Study the drawing (mm; zero at the part's minimum x, y, z) and answer. A direction names the side the tool comes from. Round coordinates to 2 decimals unless told otherwise and drop trailing zeros. Order: outer loops, then holes, each group sorted by start corner. A loop starts at its lowest first (then second) coordinate and runs counter-clockwise, first axis right, second up. Notation, with made-up numbers: (-36.75, 32) -> (-8.75, 32) arc R19 cw to (-8.75, 37) -> close; hole circle Ø9 at (62, 22). An arc over 180 degrees is marked (long way). Use one line per item in the form item = value.
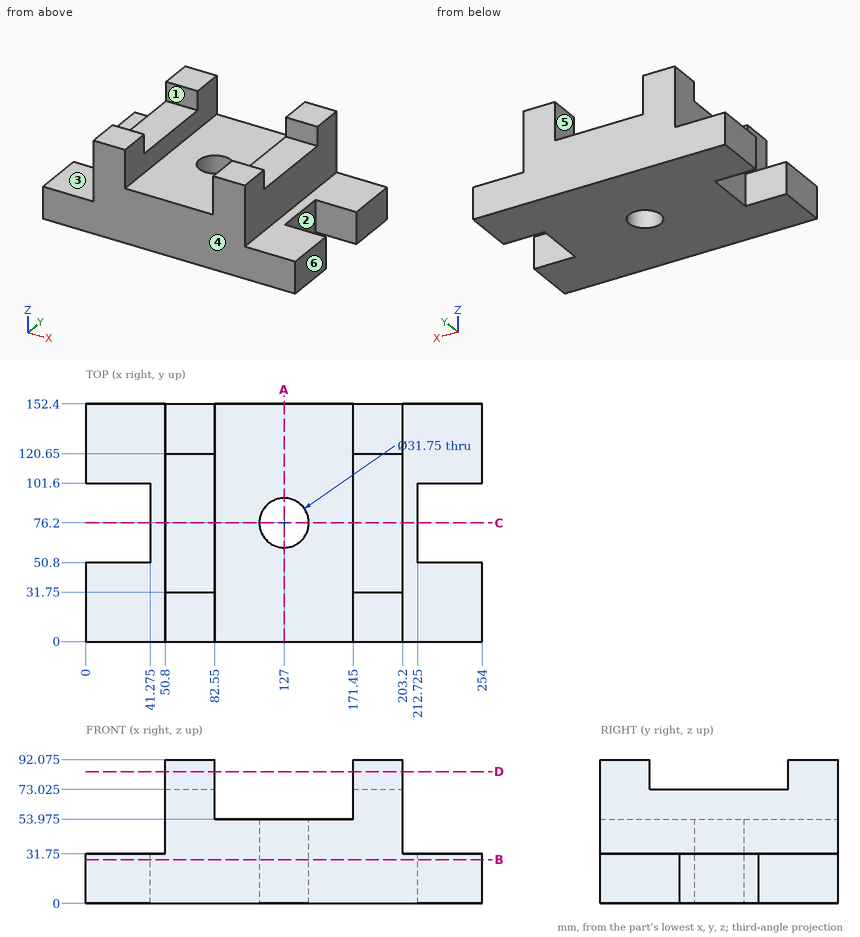
Item 1: Flat-ended cylindrical pins translate along their axes: P1, Ø1, axis at y = 120, z = 66.5, coming from the -X side; P2, Ø3, axis at x = 213.5, y = 68.5, coming from the -Z side; P3, Ø8, axis at y = 33.5, z = 81, coming from the +X side; P4, Ø5, axis at y = 77.5, z = 21, coming from the +X side (3 decimals). Find the tip coordinate at first contact, or state that the pin passes through.
Findings:
P1 = 50.8
P2 = 0
P3 = 203.2
P4 = 212.725
Item 2: For the marked faces 1, 2 and 3, determine the directions among +Z, -Z, +X, -X, +Y, -Y from which every point of the face is accessible in a straight line to the end or side of a thin tool.
Findings:
face_1 = +Z, +X, -X
face_2 = +Z, -Z, +X
face_3 = +Z, -X, +Y, -Y
Item 3: Consider line 1 along Y through (x, z) = (127, 38) (3 decimals); line 2 along X through (y, z) = (144.5, 62); line 3 along Y through (x, z) = (225.5, 26.5). Determine where each line is inside the solid, lowest interval first.
Findings:
line_1 = 0 to 60.325, 92.075 to 152.4
line_2 = 50.8 to 82.55, 171.45 to 203.2
line_3 = 0 to 50.8, 101.6 to 152.4
Item 4: The part is cut by section B-B, the plane z = 28. Give the vertices of the cut face in (x, y) (3 decimals).
Findings:
outline = (0, 0) -> (254, 0) -> (254, 50.8) -> (212.725, 50.8) -> (212.725, 101.6) -> (254, 101.6) -> (254, 152.4) -> (0, 152.4) -> (0, 101.6) -> (41.275, 101.6) -> (41.275, 50.8) -> (0, 50.8) -> close; hole circle Ø31.75 at (127, 76.2)
Item 5: The part is cut by section C-C, the plane y = 76.2. Give the vertices of the cut face in (x, z) (3 decimals), and give its area (3 significant figures).
Findings:
outline = (41.275, 0) -> (111.125, 0) -> (111.125, 53.975) -> (82.55, 53.975) -> (82.55, 73.025) -> (50.8, 73.025) -> (50.8, 31.75) -> (41.275, 31.75) -> close; (142.875, 0) -> (212.725, 0) -> (212.725, 31.75) -> (203.2, 31.75) -> (203.2, 73.025) -> (171.45, 73.025) -> (171.45, 53.975) -> (142.875, 53.975) -> close
area = 8,330 mm^2
Item 6: The part is cut by section D-D, the plane z = 84.5. Give the vertices of the cut face in (x, y), and give its area (3 significant figures).
Findings:
outline = (50.8, 0) -> (82.55, 0) -> (82.55, 31.75) -> (50.8, 31.75) -> close; (50.8, 120.65) -> (82.55, 120.65) -> (82.55, 152.4) -> (50.8, 152.4) -> close; (171.45, 0) -> (203.2, 0) -> (203.2, 31.75) -> (171.45, 31.75) -> close; (171.45, 120.65) -> (203.2, 120.65) -> (203.2, 152.4) -> (171.45, 152.4) -> close
area = 4,030 mm^2
Item 7: The part is cut by section A-A, the plane x = 127. Give the vertices of the cut face in (y, z) (3 decimals).
Findings:
outline = (0, 0) -> (60.325, 0) -> (60.325, 53.975) -> (0, 53.975) -> close; (92.075, 0) -> (152.4, 0) -> (152.4, 53.975) -> (92.075, 53.975) -> close
Item 8: Determine the mould class of the marked faces 4, 5 and 6 for opening direction X: released by +X, released by -X, zero draft, split by the parting line, or undercut.
Findings:
face_4 = zero draft
face_5 = undercut
face_6 = released by +X
